from build123d import *

# Parameters (mm, degrees)
F1_DEPTH = 20
F2_R     = 2
F3_R     = 4
F4_R     = 5
F5_DEPTH = 0.01


with BuildPart() as f1:
    # F0 (on Top) → F1 (new body, symmetric)
    with BuildSketch(Plane.XY):
        Polygon((137.5, 0), (0, 0), (-137.5, 0), (-137.5, -25), (-117.5, -25), (-117.5, -23), (-135.5, -23), (-135.5, -2), (0, -2), (135.5, -2), (135.5, -23), (117.5, -23), (117.5, -25), (137.5, -25), align=None)
    extrude(amount=F1_DEPTH, both=True)

    # F2
    f2_edges = [f1.edges().sort_by_distance(p)[0] for p in [
        (-135.5, -23, 0),
        (-135.5, -2, 0),
        (135.5, -23, 0),
        (135.5, -2, 0),
    ]]
    fillet(f2_edges, radius=F2_R)

    # F3
    f3_edges = [f1.edges().sort_by_distance(p)[0] for p in [
        (-137.5, -25, 0),
        (-137.5, 0, 0),
        (137.5, -25, 0),
        (137.5, 0, 0),
    ]]
    fillet(f3_edges, radius=F3_R)

    # F4 (on face) → F5 (cut)
    with BuildSketch(Plane.XZ.offset(2)):
        with Locations((0, 13)):
            Circle(F4_R)
    extrude(amount=-F5_DEPTH, mode=Mode.SUBTRACT)


solid = f1.part
Here's how the part is built. I have some questions about the finished solid (model axes, mm). A direction names the side the tool comes from. Coordinates: 2 decimals unless noted, no trailing zeros. Write each loop counter-clockwise with the first axis right and the second up, starting at its lowest first coordinate (ties: lowest second). Pieces come first, ordered by that corner, then holes.
Item 1: On a 3-axis mill with a long thin cutter (end or side, diameter ignored), from which of +Z, -Z, +X, -X, +Y, -Y can I reach the whole of each face in a straight line? I mean faces 5 (the flat face through (-135.5, -13, 0)), 6 (the flat face through (2, 0, 0)), 7 (the flat face through (0, -1.99, 13)). Say none if no direction works.
Item 2: If we mould it in two halves opening along X, with no side actions, what happens to faces 1 (the flat face through (-126, -25, 0)), 2 (the flat face through (135.5, -12, 0)), 3 (the flat face through (137.5, -13, 0)), 4 (the flat face through (-137.5, -12, 0))? For each: +X half, -X half, draft (parallel to the pull), parting line (faces both ways), or undercut.
Item 3: Will these pins go through, and if not, where does the flat tip stop? pin 1 (0.6 mm diameter, centred on y = -24, z = 8.5, fed in from -X); pin 2 (20 mm diameter, centred on x = -36.5, z = -7, fed in from -Y); pin 3 (1 mm diameter, centred on y = -24, z = -2, fed in from +X).
Item 4: If I drill on line 1 (Y direction, x = 120.5, z = 6.5); line 2 (X direction, y = -17.75, z = -2); line 3 (Y direction, x = -75, z = 9), over which ranges is the centre line in solid material (lowest first)?
Item 5: I want a section at B-B on z = -16. Write out the boundary of the cut face in (x, y).
Item 6: I want a section at A-A on y = -16.75. Write out the boundary of the cut face in (x, z).
Findings below:
1. face 5: +Z, -Z
1. face 6: +Z, -Z, +X, -X, +Y
1. face 7: +Z, -Z, -Y
2. face 1: draft
2. face 2: undercut
2. face 3: +X half
2. face 4: -X half
3. pin 1: stops at x = -136.45
3. pin 2: stops at y = -2
3. pin 3: stops at x = 136.62
4. line 1: y = -25 to -23, -2 to 0
4. line 2: x = -137.5 to -135.5, 135.5 to 137.5
4. line 3: y = -2 to 0
5. outline: (-137.5, -21) arc R4 ccw to (-133.5, -25) - (-117.5, -25) - (-117.5, -23) - (-133.5, -23) arc R2 cw to (-135.5, -21) - (-135.5, -4) arc R2 cw to (-133.5, -2) - (133.5, -2) arc R2 cw to (135.5, -4) - (135.5, -21) arc R2 cw to (133.5, -23) - (117.5, -23) - (117.5, -25) - (133.5, -25) arc R4 ccw to (137.5, -21) - (137.5, -4) arc R4 ccw to (133.5, 0) - (-133.5, 0) arc R4 ccw to (-137.5, -4) - close
6. outline: (-137.5, -20) - (-135.5, -20) - (-135.5, 20) - (-137.5, 20) - close; (135.5, -20) - (137.5, -20) - (137.5, 20) - (135.5, 20) - close
